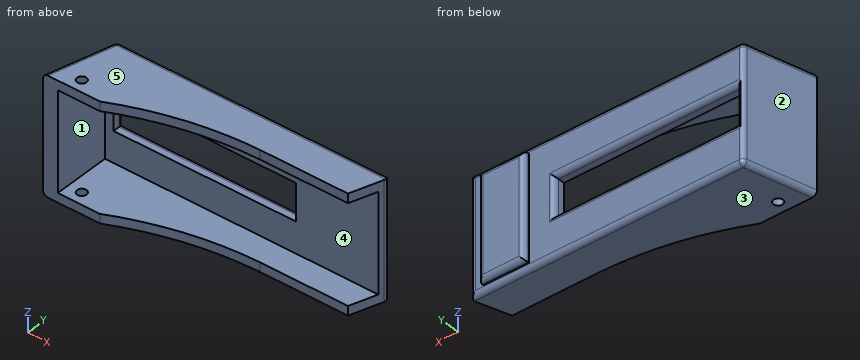
from build123d import *

# Parameters (mm, degrees)
SKETCH5_W           = 53.848
SKETCH5_H           = 14.0335
SKETCH5_W_2         = 9.3472
SKETCH5_H_2         = 1.27
BOSS_EXTRUDE2_DEPTH = 24.13
SKETCH7_R           = 0.97155
CUT_EXTRUDE3_DEPTH  = 40.748679545
SKETCH8_W           = 9.3472
SKETCH8_H           = 1.27
CUT_EXTRUDE4_DEPTH  = 1.27
SKETCH9_W           = 37.465
SKETCH9_H           = 7.62
CUT_EXTRUDE5_DEPTH  = 42.33069605
SKETCH10_W          = 56.896
SKETCH10_H          = 20.32
CUT_EXTRUDE6_DEPTH  = 11.684
FILLET1_R           = 1.016
FILLET5_R           = 1.016


with BuildPart() as part:
    # Sketch5 → Boss-Extrude2 (new body)
    with BuildSketch(Plane.XY):
        Rectangle(SKETCH5_W, SKETCH5_H)
        Polygon((26.924, 7.01675), (26.924, -0.71755), (29.464, 7.01675), align=None)
        Polygon((-26.924, 7.01675), (-30.48, -7.01675), (-26.924, -7.01675), align=None)
        with Locations((21.7424, 7.65175)):
            Rectangle(SKETCH5_W_2, SKETCH5_H_2)
    extrude(amount=BOSS_EXTRUDE2_DEPTH)

    # Sketch7 → Cut-Extrude3 (cut, through all)
    with BuildSketch(Plane.XY.offset(24.13)):
        with BuildLine():
            Line((26.924, -7.01675), (26.924, -0.71755))
            Line((26.924, -0.71755), (8.862620223, -0.71755))
            add(Edge.make_bspline(
                [(-18.7706, -7.01675), (-5.778401918, -0.891302623), (8.862620223, -0.71755)],
                knots=[0, 0, 0, 1, 1, 1], degree=2))
            Line((-18.7706, -7.01675), (26.924, -7.01675))
        make_face()
        with Locations((-24.6126, -4.47675)):
            Circle(SKETCH7_R)
    extrude(amount=-CUT_EXTRUDE3_DEPTH, mode=Mode.SUBTRACT)

    # Sketch8 → Cut-Extrude4 (cut)
    with BuildSketch(Plane(origin=(0, 8.28675, 0), x_dir=(1, 0, 0), z_dir=(0, 1, 0))):
        with Locations((21.7424, -0.635)):
            Rectangle(SKETCH8_W, SKETCH8_H)
        with Locations((21.7424, -23.495)):
            Rectangle(SKETCH8_W, SKETCH8_H)
    extrude(amount=-CUT_EXTRUDE4_DEPTH, mode=Mode.SUBTRACT)

    # Sketch9 → Cut-Extrude5 (cut, through all)
    with BuildSketch(Plane(origin=(0, 7.01675, 0), x_dir=(1, 0, 0), z_dir=(0, 1, 0))):
        with Locations((-6.9215, -12.065)):
            Rectangle(SKETCH9_W, SKETCH9_H)
    extrude(amount=-CUT_EXTRUDE5_DEPTH, mode=Mode.SUBTRACT)

    # Sketch10 → Cut-Extrude6 (cut)
    with BuildSketch(Plane.XZ.offset(7.01675)):
        with Locations((1.016, 12.065)):
            Rectangle(SKETCH10_W, SKETCH10_H)
    extrude(amount=-CUT_EXTRUDE6_DEPTH, mode=Mode.SUBTRACT)

    # Fillet1
    # the kernel refuses this fillet: 1.016 mm, written as the material it takes off along each edge
    with BuildSketch(Plane(origin=(-26.133337543, 6.00075, 1.016), x_dir=(-0.9693635135141576, 0.2456305735601486, 0), z_dir=(0, 0, -1))) as fillet1_piece_1_section:
        Polygon((0, 0), (FILLET1_R, 0), (FILLET1_R, FILLET1_R * 0.778211079665), (FILLET1_R * 0.24563057356, FILLET1_R * 0.969363513514), align=None)
    fillet1_piece_1 = extrude(amount=FILLET1_R, mode=Mode.PRIVATE)
    fillet1_piece_1 = fillet1_piece_1 - Plane(origin=(-26.133337543, 6.00075, 1.016), x_dir=(0.6141536560339975, -0.7891864714882498, 0), z_dir=(0, 0, -1)) * Sphere(FILLET1_R, mode=Mode.PRIVATE)
    add(fillet1_piece_1, mode=Mode.SUBTRACT)
    with BuildSketch(Plane(origin=(-26.133337543, 6.00075, 23.114), x_dir=(-0.9693635135141576, 0.2456305735601486, 0), z_dir=(0, 0, 1))) as fillet1_piece_2_section:
        Polygon((0, 0), (FILLET1_R, 0), (FILLET1_R, -FILLET1_R * 0.778211079665), (FILLET1_R * 0.24563057356, -FILLET1_R * 0.969363513514), align=None)
    fillet1_piece_2 = extrude(amount=FILLET1_R, mode=Mode.PRIVATE)
    fillet1_piece_2 = fillet1_piece_2 - Plane(origin=(-26.133337543, 6.00075, 23.114), x_dir=(0.6141536560339975, -0.7891864714882498, 0), z_dir=(0, 0, 1)) * Sphere(FILLET1_R, mode=Mode.PRIVATE)
    add(fillet1_piece_2, mode=Mode.SUBTRACT)
    with BuildSketch(Plane(origin=(-26.924, 7.01675, 1.016), x_dir=(-0.24563057356014745, -0.969363513514158, 0), z_dir=(0, 0, 1))) as fillet1_piece_3:
        with BuildLine():
            CenterArc((FILLET1_R * 0.778211079665, FILLET1_R), FILLET1_R, 194.219101718, 75.780898282)
            Line((-FILLET1_R * 0.191152433849, FILLET1_R * 0.75436942644), (0, 0))
            Line((0, 0), (FILLET1_R * 0.778211079665, 0))
        make_face()
    extrude(amount=22.098, mode=Mode.SUBTRACT)
    with BuildSketch(Plane(origin=(29.464, 7.01675, -3.507619048), x_dir=(-0.312012480499221, -0.9500780031201245, 0), z_dir=(0, 0, 1))) as fillet1_piece_4:
        with BuildLine():
            CenterArc((FILLET1_R * 1.38095238095, -FILLET1_R), FILLET1_R, 90, 108.180553842)
            Line((FILLET1_R * 0.430874377832, -FILLET1_R * 1.3120124805), (0, 0))
            Line((0, 0), (FILLET1_R * 1.38095238095, 0))
        make_face()
    extrude(amount=31.145238095, mode=Mode.SUBTRACT)
    with BuildSketch(Plane(origin=(32.004, 7.01675, 24.13), x_dir=(0, -1, 0), z_dir=(-1, 0, 0)), Plane(origin=(-26.133337543, 7.01675, 0), x_dir=(0, -1, 0), z_dir=(1, 0, 0))) as fillet1_piece_5:
        with BuildLine():
            CenterArc((FILLET1_R, -FILLET1_R), FILLET1_R, 90, 90)
            Line((0, -FILLET1_R), (0, 0))
            Line((0, 0), (FILLET1_R, 0))
        make_face()
    extrude(amount=58.137337543, mode=Mode.SUBTRACT)
    with BuildSketch(Plane(origin=(-27.118210873, 6.250310663, 24.13), x_dir=(0.9693635135141576, -0.24563057356014859, -3.4967654318902577e-15), z_dir=(-0.2456305735601486, -0.9693635135141576, 0)), Plane(origin=(-27.118210873, 6.250310663, 0), x_dir=(0, 0, 1), z_dir=(-0.2456305735601486, -0.9693635135141576, 0))) as fillet1_piece_6:
        with BuildLine():
            CenterArc((FILLET1_R, -FILLET1_R), FILLET1_R, 90, 90)
            Line((0, -FILLET1_R), (0, 0))
            Line((0, 0), (FILLET1_R, 0))
        make_face()
    extrude(amount=16.22636273, mode=Mode.SUBTRACT)
    with BuildSketch(Plane(origin=(11.811, 7.01675, 15.875), x_dir=(1, 0, 0), z_dir=(0, 0, -1)), Plane(origin=(-25.654, 7.01675, 8.255), x_dir=(-1, 0, 0), z_dir=(0, 0, 1))) as fillet1_piece_7:
        with BuildLine():
            CenterArc((FILLET1_R, FILLET1_R), FILLET1_R, 180, 90)
            Line((0, FILLET1_R), (0, 0))
            Line((0, 0), (FILLET1_R, 0))
        make_face()
    extrude(amount=7.62, mode=Mode.SUBTRACT)
    with BuildSketch(Plane(origin=(11.811, 7.01675, 8.255), x_dir=(0, 0, -1), z_dir=(-1, 0, 0)), Plane(origin=(-25.654, 7.01675, 15.875), x_dir=(0, 0, 1), z_dir=(1, 0, 0))) as fillet1_piece_8:
        with BuildLine():
            CenterArc((FILLET1_R, FILLET1_R), FILLET1_R, 180, 90)
            Line((0, FILLET1_R), (0, 0))
            Line((0, 0), (FILLET1_R, 0))
        make_face()
    extrude(amount=37.465, mode=Mode.SUBTRACT)
    with BuildSketch(Plane(origin=(11.811, 7.01675, 18.415), x_dir=(1, 0, 0), z_dir=(0, 0, -1))) as fillet1_piece_9a_section:
        with BuildLine():
            CenterArc((FILLET1_R, FILLET1_R), FILLET1_R, 180, 90)
            Line((0, FILLET1_R), (0, 0))
            Line((0, 0), (FILLET1_R, 0))
        make_face()
    fillet1_piece_9a = extrude(amount=10.16, mode=Mode.PRIVATE)
    fillet1_piece_9a = split(fillet1_piece_9a, bisect_by=Plane(origin=(12.041017436, 6.786732564, 15.875), z_dir=(0, 0, 1)), keep=Keep.TOP, mode=Mode.PRIVATE)
    with BuildSketch(Plane(origin=(-25.654, 7.01675, 15.875), x_dir=(0, 0, 1), z_dir=(1, 0, 0))) as fillet1_piece_9b_section:
        with BuildLine():
            CenterArc((FILLET1_R, FILLET1_R), FILLET1_R, 180, 90)
            Line((0, FILLET1_R), (0, 0))
            Line((0, 0), (FILLET1_R, 0))
        make_face()
    fillet1_piece_9b = extrude(amount=40.005, mode=Mode.PRIVATE)
    fillet1_piece_9b = split(fillet1_piece_9b, bisect_by=Plane(origin=(11.811, 6.786732564, 16.105017436), z_dir=(1, 0, 0)), keep=Keep.TOP, mode=Mode.PRIVATE)
    fillet1_piece_9 = fillet1_piece_9a & fillet1_piece_9b
    add(fillet1_piece_9, mode=Mode.SUBTRACT)
    with BuildSketch(Plane(origin=(14.351, 7.01675, 8.255), x_dir=(0, 0, -1), z_dir=(-1, 0, 0))) as fillet1_piece_10a_section:
        with BuildLine():
            CenterArc((FILLET1_R, FILLET1_R), FILLET1_R, 180, 90)
            Line((0, FILLET1_R), (0, 0))
            Line((0, 0), (FILLET1_R, 0))
        make_face()
    fillet1_piece_10a = extrude(amount=40.005, mode=Mode.PRIVATE)
    fillet1_piece_10a = split(fillet1_piece_10a, bisect_by=Plane(origin=(11.811, 6.786732564, 8.024982564), z_dir=(1, 0, 0)), keep=Keep.TOP, mode=Mode.PRIVATE)
    with BuildSketch(Plane(origin=(11.811, 7.01675, 15.875), x_dir=(1, 0, 0), z_dir=(0, 0, -1))) as fillet1_piece_10b_section:
        with BuildLine():
            CenterArc((FILLET1_R, FILLET1_R), FILLET1_R, 180, 90)
            Line((0, FILLET1_R), (0, 0))
            Line((0, 0), (FILLET1_R, 0))
        make_face()
    fillet1_piece_10b = extrude(amount=10.16, mode=Mode.PRIVATE)
    fillet1_piece_10b = split(fillet1_piece_10b, bisect_by=Plane(origin=(12.041017436, 6.786732564, 8.255), z_dir=(0, 0, -1)), keep=Keep.TOP, mode=Mode.PRIVATE)
    fillet1_piece_10 = fillet1_piece_10a & fillet1_piece_10b
    add(fillet1_piece_10, mode=Mode.SUBTRACT)
    with BuildSketch(Plane(origin=(-25.654, 7.01675, 5.715), x_dir=(-1, 0, 0), z_dir=(0, 0, 1))) as fillet1_piece_11a_section:
        with BuildLine():
            CenterArc((FILLET1_R, FILLET1_R), FILLET1_R, 180, 90)
            Line((0, FILLET1_R), (0, 0))
            Line((0, 0), (FILLET1_R, 0))
        make_face()
    fillet1_piece_11a = extrude(amount=10.16, mode=Mode.PRIVATE)
    fillet1_piece_11a = split(fillet1_piece_11a, bisect_by=Plane(origin=(-25.884017436, 6.786732564, 8.255), z_dir=(0, 0, -1)), keep=Keep.TOP, mode=Mode.PRIVATE)
    with BuildSketch(Plane(origin=(11.811, 7.01675, 8.255), x_dir=(0, 0, -1), z_dir=(-1, 0, 0))) as fillet1_piece_11b_section:
        with BuildLine():
            CenterArc((FILLET1_R, FILLET1_R), FILLET1_R, 180, 90)
            Line((0, FILLET1_R), (0, 0))
            Line((0, 0), (FILLET1_R, 0))
        make_face()
    fillet1_piece_11b = extrude(amount=40.005, mode=Mode.PRIVATE)
    fillet1_piece_11b = split(fillet1_piece_11b, bisect_by=Plane(origin=(-25.654, 6.786732564, 8.024982564), z_dir=(-1, 0, 0)), keep=Keep.TOP, mode=Mode.PRIVATE)
    fillet1_piece_11 = fillet1_piece_11a & fillet1_piece_11b
    add(fillet1_piece_11, mode=Mode.SUBTRACT)
    with BuildSketch(Plane(origin=(-25.654, 7.01675, 8.255), x_dir=(-1, 0, 0), z_dir=(0, 0, 1))) as fillet1_piece_12a_section:
        with BuildLine():
            CenterArc((FILLET1_R, FILLET1_R), FILLET1_R, 180, 90)
            Line((0, FILLET1_R), (0, 0))
            Line((0, 0), (FILLET1_R, 0))
        make_face()
    fillet1_piece_12a = extrude(amount=10.16, mode=Mode.PRIVATE)
    fillet1_piece_12a = split(fillet1_piece_12a, bisect_by=Plane(origin=(-25.884017436, 6.786732564, 15.875), z_dir=(0, 0, 1)), keep=Keep.TOP, mode=Mode.PRIVATE)
    with BuildSketch(Plane(origin=(-28.194, 7.01675, 15.875), x_dir=(0, 0, 1), z_dir=(1, 0, 0))) as fillet1_piece_12b_section:
        with BuildLine():
            CenterArc((FILLET1_R, FILLET1_R), FILLET1_R, 180, 90)
            Line((0, FILLET1_R), (0, 0))
            Line((0, 0), (FILLET1_R, 0))
        make_face()
    fillet1_piece_12b = extrude(amount=40.005, mode=Mode.PRIVATE)
    fillet1_piece_12b = split(fillet1_piece_12b, bisect_by=Plane(origin=(-25.654, 6.786732564, 16.105017436), z_dir=(-1, 0, 0)), keep=Keep.TOP, mode=Mode.PRIVATE)
    fillet1_piece_12 = fillet1_piece_12a & fillet1_piece_12b
    add(fillet1_piece_12, mode=Mode.SUBTRACT)

    # Fillet5
    fillet5_edges = [part.edges().sort_by_distance(p)[0] for p in [
        (26.416, 8.28675, 12.065),
        (17.0688, 8.28675, 12.065),
        (21.7424, 8.28675, 1.27),
        (21.7424, 8.28675, 22.86),
    ]]
    fillet(fillet5_edges, radius=FILLET5_R)


solid = part.part
Could you check a few things on this model? Use its own coordinates, in mm. Face numbers are marked on the shaded views. A direction names the side the tool comes from. Coordinates: 2 decimals unless noted, no trailing zeros. Order: outer loops, then holes, each group sorted by start corner. A loop starts at its lowest first (then second) coordinate and runs counter-clockwise, first axis right, second up. Notation, with made-up numbers: (67, 37.25) - (92, 37.25) arc R29 ccw to (92, 72.25) - close; hole circle Ø6 at (-22, 41.5). An arc over 180 degrees is marked (long way). Answer in a Markdown table with one row per item. Add a question column.
(1) I need wall thicknesses on L1, parallel to Z at x = -4.5, y = 1.5 (3 decimals); L2, parallel to Z at x = 3.5, y = 5.25 (3 decimals); L3, parallel to Y at x = 1.5, z = 18.75. Which ranges of each line are inside material? Lowest first, please.
(2) If we mould it in two halves opening along Z, with no side actions, what happens to the marked faces 3, 4 and 5? For each: released by +Z, released by -Z, zero draft, split by the parting line, or undercut.
(3) If we section it at A-A, the plane x = 16.5: Please give me the cut outline in (y, z) (3 decimals), then the cut area to 3 significant figures.
(4) Will these pins go through, and if not, where does the flat tip stop? pin 1 (0.7 mm diameter, centred on y = 5.5, z = 13.5, fed in from -X); pin 2 (11 mm diameter, centred on x = 12.5, z = 8.5, fed in from +Y); pin 3 (1.5 mm diameter, centred on y = 3, z = 17, fed in from -X); pin 4 (1.7 mm diameter, centred on x = -24.61, y = -4.48, fed in from -Z).
(5) If we section it at B-B, the plane z = 3.25: Please give me the cut outline in (x, y).
(6) On a 3-axis mill with a long thin cutter (end or side, diameter ignored), from which of +Z, -Z, +X, -X, +Y, -Y can I reach the whole of each face in a straight line? I mean the marked faces 1 and 2. Say none if no direction works.
Results are:
| question | item | result |
|---|---|---|
| 1 | L1 | z = 0 to 1.905, 22.225 to 24.13 |
| 1 | L2 | z = 0 to 8.255, 15.875 to 24.13 |
| 1 | L3 | y = 4.67 to 7.02 |
| 2 | face 3 | released by -Z |
| 2 | face 4 | undercut |
| 2 | face 5 | released by +Z |
| 3 | outline | (-0.718, 0) - (6.001, 0) arc R1.016 ccw to (7.017, 1.016) - (7.017, 23.114) arc R1.016 ccw to (6.001, 24.13) - (-0.718, 24.13) - (-0.718, 22.225) - (4.667, 22.225) - (4.667, 1.905) - (-0.718, 1.905) - close |
| 3 | area | 76.8 mm2 |
| 4 | pin 1 | stops at x = -27.4 |
| 4 | pin 2 | stops at y = 8.28 |
| 4 | pin 3 | stops at x = -28.13 |
| 4 | pin 4 | passes through |
| 5 | outline | (-30.48, -7.02) - (-27.43, -7.02) - (-27.43, 4.67) - (28.69, 4.67) - (29.03, 5.68) arc R1.02 ccw to (28.06, 7.02) - (26.42, 7.02) - (26.42, 7.27) arc R1.02 ccw to (25.4, 8.29) - (18.08, 8.29) arc R1.02 ccw to (17.07, 7.27) - (17.07, 7.02) - (-26.13, 7.02) arc R1.02 ccw to (-27.12, 6.25) - close |
| 6 | face 1 | +X, -Y |
| 6 | face 2 | +Z, -Z, -X, +Y |
